from build123d import *

# Parameters (mm, degrees)
SKETCH008_W  = 57.65
SKETCH008_H  = 50
PAD_DEPTH    = 23.5
SKETCH_R     = 13.15
HOLE_DEPTH   = 23.6
SKETCH009_R  = 3.015
POCKET_DEPTH = 23.501
FILLET_R     = 12


with BuildPart() as part:
    # Sketch008 → Pad (new body)
    with BuildSketch(Plane.XY):
        with Locations((3.825, 0)):
            Rectangle(SKETCH008_W, SKETCH008_H)
    extrude(amount=PAD_DEPTH)

    # Sketch (on Face6 of Pad) → Hole (cut)
    with BuildSketch(Plane.XY.offset(23.5)):
        Circle(SKETCH_R)
    extrude(amount=-HOLE_DEPTH, mode=Mode.SUBTRACT)

    # Sketch009 (on Face5 of Hole) → Pocket (cut, through all)
    with BuildSketch(Plane.XY.offset(23.5)):
        with Locations((-16, 8.955)):
            Circle(SKETCH009_R)
        with Locations((-16, -8.955)):
            Circle(SKETCH009_R)
        with Locations((16, 8.955)):
            Circle(SKETCH009_R)
        with Locations((16, -8.955)):
            Circle(SKETCH009_R)
    extrude(amount=-POCKET_DEPTH, mode=Mode.SUBTRACT)

    # Fillet
    fillet_edges = [part.edges().sort_by_distance(p)[0] for p in [
        (-25, 25, 11.75),
        (-25, -25, 11.75),
    ]]
    fillet(fillet_edges, radius=FILLET_R)


solid = part.part
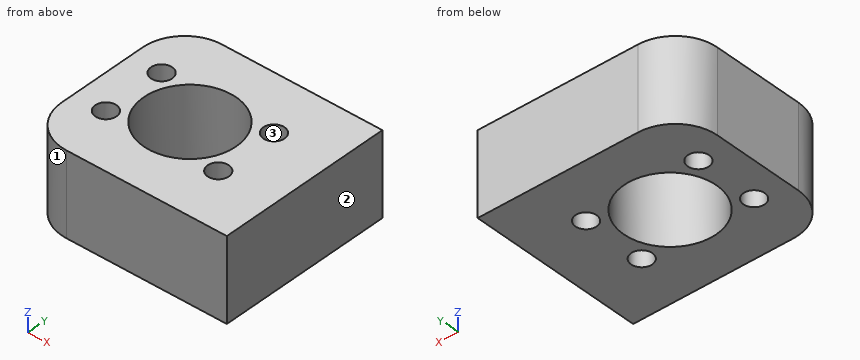
Could you check a few things on this model? Use its own coordinates, in mm. Face numbers are marked on the shaded views. Round coordinates to 2 decimals unless told otherwise and drop trailing zeros. Write each loop counter-clockwise with the first axis right and the second up, starting at its lowest first coordinate (ties: lowest second). Pieces come first, ordered by that corner, then holes. Notation, with made-up numbers: (-39, 6) - (-5, 6) arc R19 ccw to (-5, 28) - close; hole circle Ø9 at (27, -1.5). An arc over 180 degrees is marked (long way). Use a Markdown table: item, result.
Q1. I want a section at B-B (y = 0). List the corners of the cut face in (x, z) for me.
Output values:
| item | result |
|---|---|
| outline | (-25, 0) - (-13.15, 0) - (-13.15, 23.5) - (-25, 23.5) - close; (13.15, 0) - (32.65, 0) - (32.65, 23.5) - (13.15, 23.5) - close |
Q2. I want a section at D-D (z = 10.5). List the corners of the cut face in (x, y) for me (3 decimals), plus the area to 3 significant figures.
Output values:
| item | result |
|---|---|
| outline | (-25, -13) arc R12 ccw to (-13, -25) - (32.65, -25) - (32.65, 25) - (-13, 25) arc R12 ccw to (-25, 13) - close; hole circle Ø6.03 at (-16, -8.955); hole circle Ø6.03 at (-16, 8.955); hole circle Ø26.3 at (0, 0); hole circle Ø6.03 at (16, -8.955); hole circle Ø6.03 at (16, 8.955) |
| area | 2,160 mm2 |
Q3. Thinking about a two-plate mould opening in X: for the marked faces 1, 2 and 3, which applies, released by +X, released by -X, zero draft, split by the parting line, or undercut?
Output values:
| item | result |
|---|---|
| face 1 | released by -X |
| face 2 | released by +X |
| face 3 | undercut |
Q4. I want a section at A-A (x = 16). List the corners of the cut face in (y, z) for me.
Output values:
| item | result |
|---|---|
| outline | (-25, 0) - (-11.97, 0) - (-11.97, 23.5) - (-25, 23.5) - close; (-5.94, 0) - (5.94, 0) - (5.94, 23.5) - (-5.94, 23.5) - close; (11.97, 0) - (25, 0) - (25, 23.5) - (11.97, 23.5) - close |
Q5. I want a section at C-C (x = -11). List the corners of the cut face in (y, z) for me.
Output values:
| item | result |
|---|---|
| outline | (-25, 0) - (-7.21, 0) - (-7.21, 23.5) - (-25, 23.5) - close; (7.21, 0) - (25, 0) - (25, 23.5) - (7.21, 23.5) - close |
Q6. Please list where these lines run through material, in increasing order: L1, parallel to Y at x = 16, z = 9; L2, parallel to X at y = -9, z = 6.5; L3, parallel to Y at x = 0, z = 6.5.
Output values:
| item | result |
|---|---|
| L1 | -25 to -11.97, -5.94 to 5.94, 11.97 to 25 |
| L2 | -25 to -19.01, -12.99 to -9.59, 9.59 to 12.99, 19.01 to 32.65 |
| L3 | -25 to -13.15, 13.15 to 25 |
